Autodesk Inventor part; units mm, degrees
ref_plane "Work Plane1" through (0, 0, -2.5) normal (0, 0, 1) x (1, 0, 0)
ref_plane "YZ Plane" through (0, 0, 0) normal (1, 0, 0) x (0, 1, 0)
ref_plane "XZ Plane" through (0, 0, 0) normal (0, 1, 0) x (-1, 0, 0)
ref_plane "Work Plane1" through (0, 0, -2.5) normal (0, 0, 1) x (1, 0, 0)
sketch "Sketch1" plane through (0, 0, -2.5) normal (0, 0, 1) x (1, 0, 0)
  circle A0 centre (0, 0) radius 2.34
extrude "Extrusion3" add sketch "Sketch1" along normal blind 2.5
sketch "Sketch2" plane through (0, 0, 0) normal (0, 0, 1) x (1, 0, 0)
  circle A0 centre (0, 0) radius 1.25
extrude "Extrusion2" add sketch "Sketch2" along normal blind 10
sketch "Sketch3" plane through (0, 0, -2.5) normal (0, 0, 1) x (1, 0, 0)
  line L0 (0.5947, -1.03) -> (-0.5947, -1.03)
  line L1 (0.5947, 1.03) -> (1.1893, 0)
  line L2 (-0.5947, -1.03) -> (-1.1893, 0)
  line L3 (-1.1893, 0) -> (-0.5947, 1.03)
  line L4 (1.1893, 0) -> (0.5947, -1.03)
  line L5 (-0.5947, 1.03) -> (0.5947, 1.03)
extrude "Extrusion1" cut sketch "Sketch3" along normal blind 2.5
fillet "Fillet1" radius 0.1 2 edges at (-2.34, 0, 0) (-2.34, 0, -2.5)
chamfer "Chamfer1" distance 0.2 angle 45 1 edges at (-1.25, 0, 10)
properties part number "M2.5 x 10mm SHCS"
CAD build for the part. Positions are in the model's coordinates, mm. A direction names the side the tool comes from. Give positions to 0.01 mm unless a question says otherwise; leave off trailing zeros. Order: outer loops, then holes, each group sorted by start corner. A loop starts at its lowest first (then second) coordinate and runs counter-clockwise, first axis right, second up.
(1) Tool access for faces 1 (the flat face through (0, 0, 0)), 2 (the flat face through (1, 1, -2.5)), 3 (the flat face through (1, -1, 0)): list every direction of +Z, -Z, +X, -X, +Y, -Y with a clear straight run to the whole face (end or side of a thin tool).
(2) Saw through at B-B, the plane z = 4. Give the cut face in (x, y).
(3) Saw through at A-A, the plane x = 0. Give the cut face in (y, z).
(4) Flat gauge pin, fed straight in: pin 1 (2 mm diameter, centred on y = 0, z = 3.5, fed in from +X). Where does the tip first touch, or does it go through?
(5) Mould opens along X. For faces 4 (the cylindrical face through (-0.27, 1.22, 4.83)), 5 (the flat face through (0, 0, 10)), 6 (the flat face through (0.9, 0.5, -1.3)) say: released by +X, released by -X, zero draft, split by the parting line, or undercut.
(6) Drill centre lines: L1, parallel to Z at x = -1.35, y = -1.1; L2, parallel to Z at x = 0.5, y = 0.85; L3, parallel to Y at x = -0.15, z = -1.75. Where is each one in solid material? Low to high.
Results found:
1. face 1: -Z
1. face 2: -Z, +X, -X, +Y, -Y
1. face 3: +Z
2. outline: circle Ø2.5 at (0, 0)
3. outline: (-2.34, -2.4) arc R0.1 ccw to (-2.24, -2.5) - (-1.03, -2.5) - (-1.03, 0) - (1.03, 0) - (1.03, -2.5) - (2.24, -2.5) arc R0.1 ccw to (2.34, -2.4) - (2.34, -0.1) arc R0.1 ccw to (2.24, 0) - (1.25, 0) - (1.25, 9.8) - (1.05, 10) - (-1.05, 10) - (-1.25, 9.8) - (-1.25, 0) - (-2.24, 0) arc R0.1 ccw to (-2.34, -0.1) - close
4. pin 1: stops at x = 1.25
5. face 4: split by the parting line
5. face 5: zero draft
5. face 6: undercut
6. L1: z = -2.5 to 0
6. L2: z = 0 to 10
6. L3: y = -2.34 to -1.03, 1.03 to 2.34
